Work out the finished part from the listing and answer in its coordinate system (mm). A direction names the side the tool comes from. Give positions to 0.01 mm unless a question says otherwise; leave off trailing zeros. Order: outer loops, then holes, each group sorted by start corner. A loop starts at its lowest first (then second) coordinate and runs counter-clockwise, first axis right, second up. Notation, with made-up numbers: (39, -26.75) -> (44, -26.75) arc R19 cw to (44, -0.75) -> close; hole circle Ø8 at (81, 80). An arc over 180 degrees is marked (long way). Answer as CSV lines item,"result". Start each with the question number.
1. For faces 4 (the conical face through (-9.214, 21.98, 0.135)), 5 (the flat face through (-6.596, 18.379, 2.226)), 6 (the flat face through (-6.772, 18.551, 0.254)), determine the directions among +Z, -Z, +X, -X, +Y, -Y from which every point of the face is accessible in a straight line to the end or side of a thin tool.
2. A cutting plane is placed at A-A (x = 5.5). Give the vertices of the cut face in (y, z).
3. A cutting plane is placed at C-C (y = 17.5). Give the vertices of the cut face in (x, z) (3 decimals).
4. Flat-ended cylindrical pins translate along their axes: pin 1 (1 mm diameter, centred on y = 14.5, z = 3, fed in from -X); pin 2 (2 mm diameter, centred on y = 19.5, z = 3.5, fed in from -X); pin 3 (3 mm diameter, centred on x = 15.75, y = 0, fed in from -Z). Find the tip coordinate at first contact, or state that the pin passes through.
5. For a pull along Y with two mould halves and no side action, classify faces 1 (the flat face through (2, 11.5, 2)), 2 (the flat face through (-19.75, 1, 2)), 3 (the cylindrical face through (-18.547, -2.859, 2.274)) as released by +Y, released by -Y, zero draft, split by the parting line, or undercut.
6. Find the intervals of material crossed by L1, parallel to Y at x = 0, z = 2.45; L2, parallel to X at y = 13.25, z = 1.45 (3 decimals); L3, parallel to Y at x = -15.75, z = 2.15, in increasing order.
7. A cutting plane is placed at B-B (z = 1.1). Give the vertices of the cut face in (x, y) (3 decimals), then the cut area to 3 significant figures.
from build123d import *

# Parameters (mm, degrees)
F0_R     = 1.65
F1_DEPTH = 4
F2_R     = 5
F3_R     = 4
F4_SIZE  = 0.5


with BuildPart() as f1:
    # F0 (on Top) → F1 (new body)
    with BuildSketch(Plane.XY):
        Polygon((-19.75, -4), (0, -4), (19.75, -4), (19.75, 4), (9.875, 23), (0, 23), (-9.875, 23), (-19.75, 4), align=None)
        with Locations((-15.75, 0)):
            Circle(F0_R, mode=Mode.SUBTRACT)
        with Locations((15.75, 0)):
            Circle(F0_R, mode=Mode.SUBTRACT)
        Polygon((-8.075, 14.5), (-8.075, 15.7), (-8.075, 16.9), (-5.075, 19.9), (8.075, 19.9), (8.075, 15.7), (8.075, 11.5), (-5.075, 11.5), align=None, mode=Mode.SUBTRACT)
    extrude(amount=F1_DEPTH)

    # F2
    f2_edges = [f1.edges().sort_by_distance(p)[0] for p in [
        (-19.75, 4, 2),
        (-9.875, 23, 2),
        (9.875, 23, 2),
        (19.75, 4, 2),
    ]]
    fillet(f2_edges, radius=F2_R)

    # F3
    f3_edges = [f1.edges().sort_by_distance(p)[0] for p in [
        (19.75, -4, 2),
        (-19.75, -4, 2),
    ]]
    fillet(f3_edges, radius=F3_R)

    # F4
    f4_edges = [f1.edges().sort_by_distance(p)[0] for p in [
        (19.75, 1.38912, 0),
        (18.578427, -2.828427, 0),
        (19.607098, 3.965082, 0),
        (0, -4, 0),
        (15.230907, 12.694964, 0),
        (-18.578427, -2.828427, 0),
        (9.433953, 22.273712, 0),
        (-19.75, 1.38912, 0),
        (0, 23, 0),
        (-19.607098, 3.965082, 0),
        (-9.433953, 22.273712, 0),
        (-15.230907, 12.694964, 0),
        (-17.4, 0, 0),
        (14.1, 0, 0),
        (-8.075, 15.7, 0),
        (-6.575, 18.4, 0),
        (1.5, 19.9, 0),
        (8.075, 15.7, 0),
        (1.5, 11.5, 0),
        (-6.575, 13, 0),
    ]]
    chamfer(f4_edges, length=F4_SIZE)


solid = f1.part
Answer sheet:
1,face 4,"-Z, -X, +Y"
1,face 5,"+Z, -Z"
1,face 6,"-Z"
2,outline,"(-4, 0.5) -> (-3.5, 0) -> (11, 0) -> (11.5, 0.5) -> (11.5, 4) -> (-4, 4) -> close; (19.9, 0.5) -> (20.4, 0) -> (22.5, 0) -> (23, 0.5) -> (23, 4) -> (19.9, 4) -> close"
3,outline,"(-12.734, 0.5) -> (-12.17, 0) -> (-8.182, 0) -> (-7.475, 0.5) -> (-7.475, 4) -> (-12.734, 4) -> close; (8.075, 0.5) -> (8.575, 0) -> (12.17, 0) -> (12.734, 0.5) -> (12.734, 4) -> (8.075, 4) -> close"
4,pin 1,"stops at x = -14.55"
4,pin 2,"stops at x = -12.21"
4,pin 3,"passes through"
5,face 1,"undercut"
5,face 2,"zero draft"
5,face 3,"released by -Y"
6,L1,"y = -4 to 11.5, 19.9 to 23"
6,L2,"x = -14.942 to -6.825, 8.075 to 14.942"
6,L3,"y = -4 to -1.65, 1.65 to 11.7"
7,outline,"(-19.75, 0) arc R4 ccw to (-15.75, -4) -> (15.75, -4) arc R4 ccw to (19.75, 0) -> (19.75, 2.778) arc R5 ccw to (19.187, 5.084) -> (11.275, 20.306) arc R5 ccw to (6.839, 23) -> (-6.839, 23) arc R5 ccw to (-11.275, 20.306) -> (-19.187, 5.084) arc R5 ccw to (-19.75, 2.778) -> close; hole circle Ø3.3 at (-15.75, 0); hole (-8.075, 14.5) -> (-5.075, 11.5) -> (8.075, 11.5) -> (8.075, 19.9) -> (-5.075, 19.9) -> (-8.075, 16.9) -> close; hole circle Ø3.3 at (15.75, 0)"
7,area,"725 mm^2"
